The listing builds one solid part. Answer for the finished solid, in the listing's coordinates (mm). A direction names the side the tool comes from. Round coordinates to 2 decimals unless told otherwise and drop trailing zeros. Loops run counter-clockwise (first coordinate to the right, second up) from the corner with the lowest first, then second, coordinate; pieces in that order, holes last. Notation, with made-up numbers: M 60,27 L 93,27 A24 cw 93,38 Z; hole C 52.5,81 d6. An arc over 180 degrees is marked long. Put each result on its own line as item: value. Start each with the question number.
(1) Section A-A, the plane x = 0 is taken. Determine the outline of the cut face in (y, z).
(2) Flat-ended cylindrical pins translate along their axes: P1, Ø7, axis at x = 0, y = 0, coming from the -Z side; P2, Ø1.5, axis at x = 3, z = 17.5, coming from the +Y side; P3, Ø3.5, axis at y = -2.5, z = 5, coming from the -X side. Find the tip coordinate at first contact, or state that the pin passes through.
(3) Section B-B, the plane z = 8 is taken. Determine the outline of the cut face in (x, y).
(4) Section C-C, the plane y = 0 is taken. Determine the outline of the cut face in (x, z), then the cut area to 3 significant figures.
(5) Section D-D, the plane z = 93 is taken. Determine the outline of the cut face in (x, y).
(6) Determine the mould class of faces 6 (the face through (8, 0, 7)), 7 (the face through (2.285, -3.584, 12.325)), 8 (the face through (9.061, 2.854, 58.174)) for opening direction Y: released by +Y, released by -Y, zero draft, split by the parting line, or undercut.
(7) Straight lines are drawn through the part: line 1 (X direction, y = 0, z = 13.5); line 2 (X direction, y = 0, z = 5). For each, find the intervals that lie inside material, in ascending order.
(8) Which of the six approach directions +Z, -Z, +X, -X, +Y, -Y give full straight-line access (tool end or side, diameter ignored) to faces 1 (the face through (-8, 0, 7)), 2 (the face through (6.384, 0, 3)), 3 (the face through (-2, -4, 0)), 4 (the face through (0, 0, 25)), 5 (the face through (0, 0, 118))?
```python
from build123d import *

# Parameters (mm, degrees)
F0_R     = 9.5
F1_DEPTH = 118
F2_W     = 9.514893
F2_H     = 14
F2_W_2   = 10.271802
F3_DEPTH = 12.5
F4_R     = 4.25
F5_DEPTH = 25


with BuildPart() as f1:
    # F0 (on Top) → F1 (new body)
    with BuildSketch(Plane.XY):
        Circle(F0_R)
    extrude(amount=F1_DEPTH)

    # F2 (on Front) → F3 (cut, symmetric)
    with BuildSketch(Plane.XZ):
        with Locations((-11.373281, 0)):
            Rectangle(F2_W, F2_H)
        with Locations((11.520066, 0)):
            Rectangle(F2_W_2, F2_H)
    extrude(amount=F3_DEPTH, both=True, mode=Mode.SUBTRACT)

    # F4 (on face) → F5 (cut)
    with BuildSketch(Plane(origin=(0, 0, 0), x_dir=(1, 0, 0), z_dir=(0, 0, -1))):
        Circle(F4_R)
    extrude(amount=-F5_DEPTH, mode=Mode.SUBTRACT)


solid = f1.part
```
Recorded:
1. outline: M -9.5,0 L -4.25,0 L -4.25,25 L 4.25,25 L 4.25,0 L 9.5,0 L 9.5,118 L -9.5,118 Z
2. P1: stops at z = 25
2. P2: stops at y = 9.23
2. P3: stops at x = -6.62
3. outline: C 0,0 d19; hole C 0,0 d8.5
4. outline: M -9.5,7 L -6.62,7 L -6.62,0 L -4.25,0 L -4.25,25 L 4.25,25 L 4.25,0 L 6.38,0 L 6.38,7 L 9.5,7 L 9.5,118 L -9.5,118 Z
4. area: 1,990 mm²
5. outline: C 0,0 d19
6. face 6: zero draft
6. face 7: undercut
6. face 8: split by the parting line
7. line 1: x = -9.5 to -4.25, 4.25 to 9.5
7. line 2: x = -6.62 to -4.25, 4.25 to 6.38
8. face 1: -Z, -X, +Y, -Y
8. face 2: -Z, +X, +Y, -Y
8. face 3: -Z, +X, -X, +Y, -Y
8. face 4: -Z
8. face 5: +Z, +X, -X, +Y, -Y
